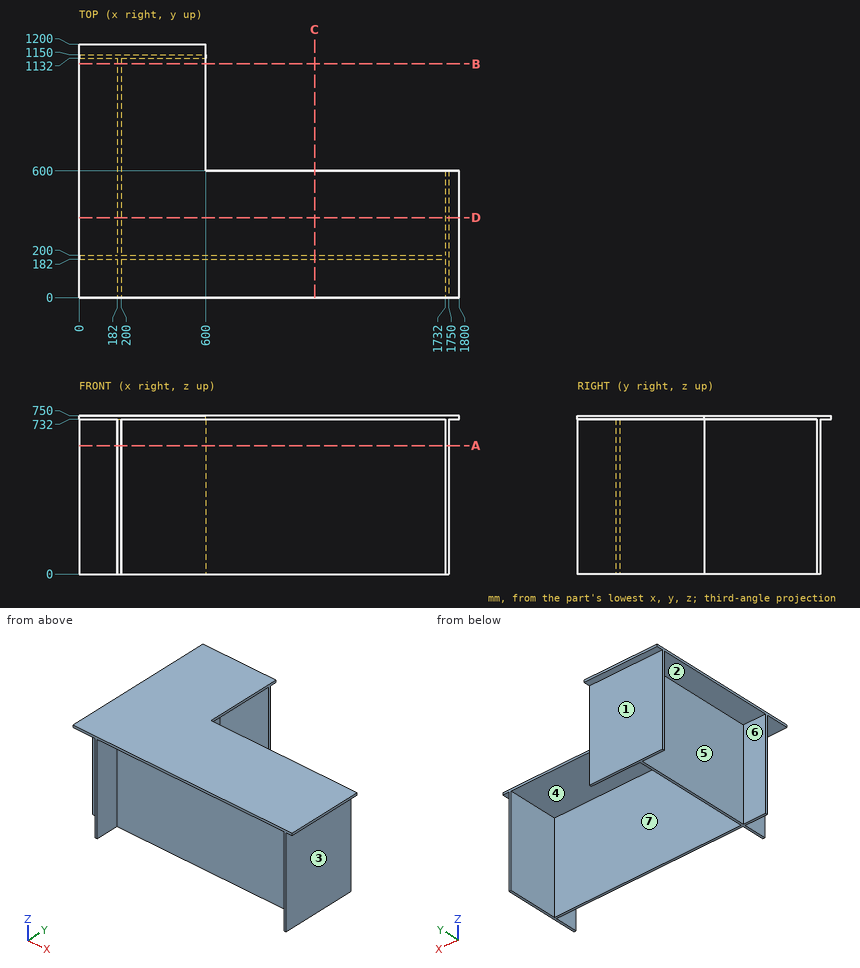
Print and shaded views of the part. All mm, measured from the part's lowest x, y and z. A direction names the side the tool comes from. Round coordinates to 2 decimals unless told otherwise and drop trailing zeros. Write each loop counter-clockwise with the first axis right and the second up, starting at its lowest first coordinate (ties: lowest second). Pieces come first, ordered by that corner, then holes. Notation, with made-up numbers: M 31.25,44 L 72.25,44 A13 ccw 72.25,64 Z; hole C -15.5,7 d3. An arc over 180 degrees is marked long. Use a Markdown table: item, result. Add a question column.
1. Drill centre lines: probe 1 along X at (y, z) = (472.5, 619); probe 2 along Y at (x, z) = (365.5, 692); probe 3 along Z at (x, y) = (407, 325). Where is each one in solid material? Low to high.
2. Flat gauge pins, fed straight in: P1, Ø15, axis at x = 1776, y = 221.5, coming from the -Z side; P2, Ø4, axis at x = 1236.5, z = 504.5, coming from the +Y side; P3, Ø6, axis at x = 845.5, z = 489.5, coming from the -Y side. Where does each tip first touch, or does it go through?
3. Slice it at B-B on y = 1106. Give the cut face in (x, z).
4. Slice it at D-D on y = 378.5. Give the cut face in (x, z).
5. Pull direction X, two halves, no side cores. Call the marked faces 4, 5, 6 and 7: released by +X, released by -X, zero draft, split by the parting line, or undercut.
6. Slice it at A-A on z = 607.5. Give the cut face in (x, y), then the cut area to 3 significant figures.
7. 3-axis set-ups, long thin cutter, end or side, ignore diameter. For the marked faces 1, 2 and 3: which of +Z, -Z, +X, -X, +Y, -Y reach the whole face in a straight line?
Reply:
| question | item | result |
|---|---|---|
| 1 | probe 1 | x = 182 to 200, 1732 to 1750 |
| 1 | probe 2 | y = 182 to 200, 1132 to 1150 |
| 1 | probe 3 | z = 732 to 750 |
| 2 | P1 | stops at z = 732 |
| 2 | P2 | stops at y = 200 |
| 2 | P3 | stops at y = 182 |
| 3 | outline | M 0,732 L 182,732 L 182,0 L 200,0 L 200,732 L 600,732 L 600,750 L 0,750 Z |
| 4 | outline | M 0,732 L 182,732 L 182,0 L 200,0 L 200,732 L 1732,732 L 1732,0 L 1750,0 L 1750,732 L 1800,732 L 1800,750 L 0,750 Z |
| 5 | face 4 | undercut |
| 5 | face 5 | released by -X |
| 5 | face 6 | zero draft |
| 5 | face 7 | undercut |
| 6 | outline | M 0,182 L 182,182 L 182,0 L 200,0 L 200,182 L 1732,182 L 1732,0 L 1750,0 L 1750,600 L 1732,600 L 1732,200 L 200,200 L 200,1132 L 600,1132 L 600,1150 L 0,1150 L 0,1132 L 182,1132 L 182,200 L 0,200 Z |
| 6 | area | 72,800 mm^2 |
| 7 | face 1 | -Z, +X, -X, +Y |
| 7 | face 2 | -Z, -X |
| 7 | face 3 | -Z, +X, +Y, -Y |
